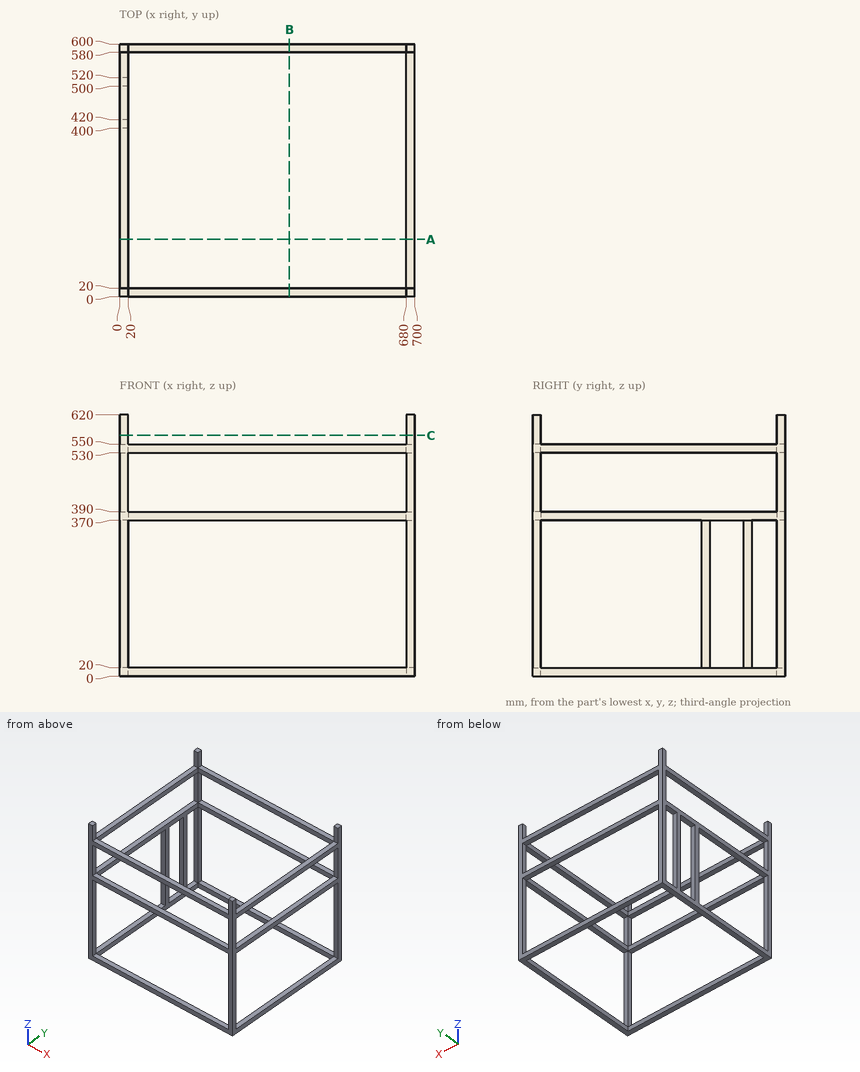
Study the drawing (mm; zero at the part's minimum x, y, z) and answer. Round coordinates to 2 decimals unless told otherwise and drop trailing zeros. Write each loop counter-clockwise with the first axis right and the second up, starting at its lowest first coordinate (ties: lowest second). Pieces come first, ordered by that corner, then holes.
1) A straight line is drawn through the part: line 1 (X direction, y = 501, z = 321). Find the intervals that lie inside material, in ascending order.
2) Given pin 1 Ø22 at (x, y) = (7.5, 327) entering from +Z, flat-ended and moving along its own axis, determine where the tip first touches the part or whether it passes through.
3) A cutting plane is placed at B-B (x = 403). Give the vertices of the cut face in (y, z).
4) A cutting plane is placed at C-C (z = 571). Give the vertices of the cut face in (x, y).
5) A cutting plane is placed at A-A (y = 136.5). Give the vertices of the cut face in (x, z).
Completed:
1. line 1: x = 0 to 20
2. pin 1: stops at z = 550
3. outline: (0, 0) - (20, 0) - (20, 20) - (0, 20) - close; (0, 370) - (20, 370) - (20, 390) - (0, 390) - close; (0, 530) - (20, 530) - (20, 550) - (0, 550) - close; (580, 0) - (600, 0) - (600, 20) - (580, 20) - close; (580, 370) - (600, 370) - (600, 390) - (580, 390) - close; (580, 530) - (600, 530) - (600, 550) - (580, 550) - close
4. outline: (0, 0) - (20, 0) - (20, 20) - (0, 20) - close; (0, 580) - (20, 580) - (20, 600) - (0, 600) - close; (680, 0) - (700, 0) - (700, 20) - (680, 20) - close; (680, 580) - (700, 580) - (700, 600) - (680, 600) - close
5. outline: (0, 0) - (20, 0) - (20, 20) - (0, 20) - close; (0, 370) - (20, 370) - (20, 390) - (0, 390) - close; (0, 530) - (20, 530) - (20, 550) - (0, 550) - close; (680, 0) - (700, 0) - (700, 20) - (680, 20) - close; (680, 370) - (700, 370) - (700, 390) - (680, 390) - close; (680, 530) - (700, 530) - (700, 550) - (680, 550) - close
